The listing builds one solid part. Answer for the finished solid, in the listing's coordinates (mm). Face numbers are marked on the shaded views. Give positions to 0.01 mm unless a question says otherwise; leave off trailing zeros. Write each loop counter-clockwise with the first axis right and the second up, starting at its lowest first coordinate (ties: lowest second). Pieces come first, ordered by that corner, then holes. Notation, with made-up numbers: (-32.5, -29) - (20.5, -29) arc R18 ccw to (20.5, -2) - close; hole circle Ø10 at (8.5, 36). An arc over 180 degrees is marked (long way). Use a Markdown table: item, result. Add a question column.
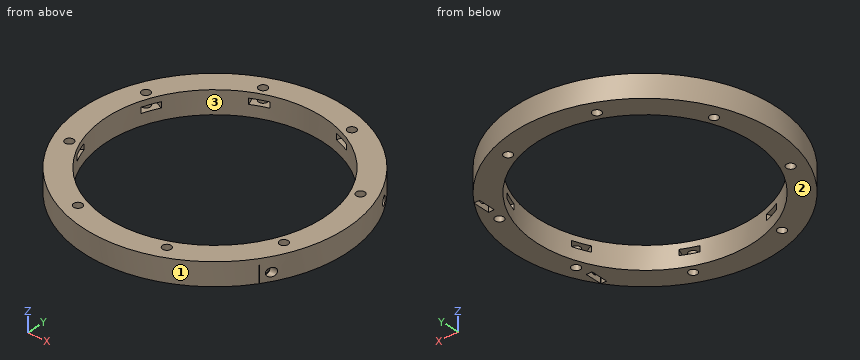
from build123d import *

# Parameters (mm, degrees)
CYLINDER1274_R               = 1.5
CYLINDER1274_DEPTH           = 60
CYLINDER1276_R               = 1.5
CYLINDER1276_DEPTH           = 60
CYLINDER1273_R               = 1.5
CYLINDER1273_DEPTH           = 60
CYLINDER1275_R               = 1.5
CYLINDER1275_DEPTH           = 60
BOX543_W                     = 2
BOX543_H                     = 6
BOX543_DEPTH                 = 6
BOX542_W                     = 2
BOX542_H                     = 6
BOX542_DEPTH                 = 6
BOX541_W                     = 2
BOX541_H                     = 6
BOX541_DEPTH                 = 6
BOX540_W                     = 2
BOX540_H                     = 6
BOX540_DEPTH                 = 6
BOX533_W                     = 8
BOX533_H                     = 6
BOX533_DEPTH                 = 2
BOX539_W                     = 8
BOX539_H                     = 6
BOX539_DEPTH                 = 2
BOX539_PLACEMENT_ANGLE       = 135
BOX534_W                     = 8
BOX534_H                     = 6
BOX534_DEPTH                 = 2
BOX536_W                     = 8
BOX536_H                     = 6
BOX536_DEPTH                 = 2
BOX536_PLACEMENT_ANGLE       = 225
BOX537_W                     = 8
BOX537_H                     = 6
BOX537_DEPTH                 = 2
BOX538_W                     = 8
BOX538_H                     = 6
BOX538_DEPTH                 = 2
BOX538_PLACEMENT_ANGLE       = 45
BOX532_W                     = 8
BOX532_H                     = 6
BOX532_DEPTH                 = 2
BOX535_W                     = 8
BOX535_H                     = 6
BOX535_DEPTH                 = 2
BOX535_PLACEMENT_ANGLE       = 45
COMPOUND921_PLACEMENT_ANGLE  = 22.5
CYLINDER1272_R               = 1.5
CYLINDER1272_DEPTH           = 60
CYLINDER1271_R               = 1.5
CYLINDER1271_DEPTH           = 60
CYLINDER1271_PLACEMENT_ANGLE = 135
CYLINDER1266_R               = 1.5
CYLINDER1266_DEPTH           = 60
CYLINDER1267_R               = 1.5
CYLINDER1267_DEPTH           = 60
CYLINDER1267_PLACEMENT_ANGLE = 225
CYLINDER1270_R               = 1.5
CYLINDER1270_DEPTH           = 60
CYLINDER1268_R               = 1.5
CYLINDER1268_DEPTH           = 60
CYLINDER1268_PLACEMENT_ANGLE = 45
CYLINDER1265_R               = 1.5
CYLINDER1265_DEPTH           = 60
CYLINDER1269_R               = 1.5
CYLINDER1269_DEPTH           = 60
CYLINDER1269_PLACEMENT_ANGLE = 45
COMPOUND919_PLACEMENT_ANGLE  = 22.5
TUBE112_R                    = 46
TUBE112_R_2                  = 38
TUBE112_DEPTH                = 8


with BuildPart() as obj1:
    # Cylinder1274 → Cylinder1274 (new body)
    with BuildSketch(Plane(origin=(32, -23, -5), x_dir=(0, 0, -1), z_dir=(1, 0, 0))):
        Circle(CYLINDER1274_R)
    extrude(amount=CYLINDER1274_DEPTH)


with BuildPart() as obj2:
    # Cylinder1276 → Cylinder1276 (new body)
    with BuildSketch(Plane(origin=(28, 51, 7), x_dir=(0, 0, -1), z_dir=(1, 0, 0))):
        Circle(CYLINDER1276_R)
    extrude(amount=CYLINDER1276_DEPTH)


with BuildPart() as obj3:
    # Cylinder1273 → Cylinder1273 (new body)
    with BuildSketch(Plane(origin=(28, -51, 7), x_dir=(0, 0, -1), z_dir=(1, 0, 0))):
        Circle(CYLINDER1273_R)
    extrude(amount=CYLINDER1273_DEPTH)


with BuildPart() as compound920:
    # Cylinder1275 → Cylinder1275 (new body)
    with BuildSketch(Plane(origin=(32, 23, -5), x_dir=(0, 0, -1), z_dir=(1, 0, 0))):
        Circle(CYLINDER1275_R)
    extrude(amount=CYLINDER1275_DEPTH)

    # Compound920: union obj1, obj2, obj3
    add(obj1.part)
    add(obj2.part)
    add(obj3.part)


with BuildPart() as krychle543:
    # Box543 → Box543 (new body)
    with BuildSketch(Plane(origin=(36, -26, -8), x_dir=(1, 0, 0), z_dir=(0, 0, 1))):
        with Locations((1, 3)):
            Rectangle(BOX543_W, BOX543_H)
    extrude(amount=BOX543_DEPTH)


with BuildPart() as krychle542:
    # Box542 → Box542 (new body)
    with BuildSketch(Plane(origin=(32, 48, 4), x_dir=(1, 0, 0), z_dir=(0, 0, 1))):
        with Locations((1, 3)):
            Rectangle(BOX542_W, BOX542_H)
    extrude(amount=BOX542_DEPTH)


with BuildPart() as krychle541:
    # Box541 → Box541 (new body)
    with BuildSketch(Plane(origin=(32, -54, 4), x_dir=(1, 0, 0), z_dir=(0, 0, 1))):
        with Locations((1, 3)):
            Rectangle(BOX541_W, BOX541_H)
    extrude(amount=BOX541_DEPTH)


with BuildPart() as compound922:
    # Box540 → Box540 (new body)
    with BuildSketch(Plane(origin=(36, 20, -8), x_dir=(1, 0, 0), z_dir=(0, 0, 1))):
        with Locations((1, 3)):
            Rectangle(BOX540_W, BOX540_H)
    extrude(amount=BOX540_DEPTH)

    # Compound922: union Krychle543, Krychle542, Krychle541
    add(krychle543.part)
    add(krychle542.part)
    add(krychle541.part)


with BuildPart() as krychle533:
    # Box533 → Box533 (new body)
    with BuildSketch(Plane(origin=(3, 37, -4), x_dir=(0, 1, 0), z_dir=(0, 0, 1))):
        with Locations((4, 3)):
            Rectangle(BOX533_W, BOX533_H)
    extrude(amount=BOX533_DEPTH)


with BuildPart() as krychle539:
    # Box539 → Box539 (new body)
    with BuildSketch(Plane.XY):
        with Locations((4, 3)):
            Rectangle(BOX539_W, BOX539_H)
    extrude(amount=BOX539_DEPTH)


with BuildPart() as krychle539_1:
    # Box539 placement: moved
    add(krychle539.part.moved(Location((-24.041631, 28.284271, -4))).rotate(Axis((-24.041631, 28.284271, -4), (0, 0, 1)), BOX539_PLACEMENT_ANGLE))


with BuildPart() as krychle534:
    # Box534 → Box534 (new body)
    with BuildSketch(Plane(origin=(-37, 3, -4), x_dir=(-1, 0, 0), z_dir=(0, 0, 1))):
        with Locations((4, 3)):
            Rectangle(BOX534_W, BOX534_H)
    extrude(amount=BOX534_DEPTH)


with BuildPart() as krychle536:
    # Box536 → Box536 (new body)
    with BuildSketch(Plane.XY):
        with Locations((4, 3)):
            Rectangle(BOX536_W, BOX536_H)
    extrude(amount=BOX536_DEPTH)


with BuildPart() as krychle536_1:
    # Box536 placement: moved
    add(krychle536.part.moved(Location((-28.284271, -24.041631, -4))).rotate(Axis((-28.284271, -24.041631, -4), (0, 0, 1)), BOX536_PLACEMENT_ANGLE))


with BuildPart() as krychle537:
    # Box537 → Box537 (new body)
    with BuildSketch(Plane(origin=(-3, -37, -4), x_dir=(0, -1, 0), z_dir=(0, 0, 1))):
        with Locations((4, 3)):
            Rectangle(BOX537_W, BOX537_H)
    extrude(amount=BOX537_DEPTH)


with BuildPart() as krychle538:
    # Box538 → Box538 (new body)
    with BuildSketch(Plane.XY):
        with Locations((4, 3)):
            Rectangle(BOX538_W, BOX538_H)
    extrude(amount=BOX538_DEPTH)


with BuildPart() as krychle538_1:
    # Box538 placement: moved
    add(krychle538.part.moved(Location((24.041631, -28.284271, -4))).rotate(Axis((24.041631, -28.284271, -4), (0, 0, -1)), BOX538_PLACEMENT_ANGLE))


with BuildPart() as krychle532:
    # Box532 → Box532 (new body)
    with BuildSketch(Plane(origin=(37, -3, -4), x_dir=(1, 0, 0), z_dir=(0, 0, 1))):
        with Locations((4, 3)):
            Rectangle(BOX532_W, BOX532_H)
    extrude(amount=BOX532_DEPTH)


with BuildPart() as compound921:
    # Box535 → Box535 (new body)
    with BuildSketch(Plane.XY):
        with Locations((4, 3)):
            Rectangle(BOX535_W, BOX535_H)
    extrude(amount=BOX535_DEPTH)


with BuildPart() as compound921_1:
    # Box535 placement: moved
    add(compound921.part.moved(Location((28.284271, 24.041631, -4))).rotate(Axis((28.284271, 24.041631, -4), (0, 0, 1)), BOX535_PLACEMENT_ANGLE))

    # Compound921: union Krychle533, Krychle539, Krychle534, Krychle536, Krychle537, Krychle538, Krychle532
    add(krychle533.part)
    add(krychle539_1.part)
    add(krychle534.part)
    add(krychle536_1.part)
    add(krychle537.part)
    add(krychle538_1.part)
    add(krychle532.part)


with BuildPart() as compound921_2:
    # Compound921 placement: moved
    add(compound921_1.part.rotate(Axis((0, 0, 0), (0, 0, 1)), COMPOUND921_PLACEMENT_ANGLE))


with BuildPart() as obj4:
    # Cylinder1272 → Cylinder1272 (new body)
    with BuildSketch(Plane(origin=(0, 41, -54), x_dir=(0, 1, 0), z_dir=(0, 0, 1))):
        Circle(CYLINDER1272_R)
    extrude(amount=CYLINDER1272_DEPTH)


with BuildPart() as obj5:
    # Cylinder1271 → Cylinder1271 (new body)
    with BuildSketch(Plane.XY):
        Circle(CYLINDER1271_R)
    extrude(amount=CYLINDER1271_DEPTH)


with BuildPart() as obj5_1:
    # Cylinder1271 placement: moved
    add(obj5.part.moved(Location((-28.991378, 28.991378, -54))).rotate(Axis((-28.991378, 28.991378, -54), (0, 0, 1)), CYLINDER1271_PLACEMENT_ANGLE))


with BuildPart() as obj6:
    # Cylinder1266 → Cylinder1266 (new body)
    with BuildSketch(Plane(origin=(-41, 0, -54), x_dir=(-1, 0, 0), z_dir=(0, 0, 1))):
        Circle(CYLINDER1266_R)
    extrude(amount=CYLINDER1266_DEPTH)


with BuildPart() as obj7:
    # Cylinder1267 → Cylinder1267 (new body)
    with BuildSketch(Plane.XY):
        Circle(CYLINDER1267_R)
    extrude(amount=CYLINDER1267_DEPTH)


with BuildPart() as obj7_1:
    # Cylinder1267 placement: moved
    add(obj7.part.moved(Location((-28.991378, -28.991378, -54))).rotate(Axis((-28.991378, -28.991378, -54), (0, 0, 1)), CYLINDER1267_PLACEMENT_ANGLE))


with BuildPart() as obj8:
    # Cylinder1270 → Cylinder1270 (new body)
    with BuildSketch(Plane(origin=(0, -41, -54), x_dir=(0, -1, 0), z_dir=(0, 0, 1))):
        Circle(CYLINDER1270_R)
    extrude(amount=CYLINDER1270_DEPTH)


with BuildPart() as obj9:
    # Cylinder1268 → Cylinder1268 (new body)
    with BuildSketch(Plane.XY):
        Circle(CYLINDER1268_R)
    extrude(amount=CYLINDER1268_DEPTH)


with BuildPart() as obj9_1:
    # Cylinder1268 placement: moved
    add(obj9.part.moved(Location((28.991378, -28.991378, -54))).rotate(Axis((28.991378, -28.991378, -54), (0, 0, -1)), CYLINDER1268_PLACEMENT_ANGLE))


with BuildPart() as obj10:
    # Cylinder1265 → Cylinder1265 (new body)
    with BuildSketch(Plane(origin=(41, 0, -54), x_dir=(1, 0, 0), z_dir=(0, 0, 1))):
        Circle(CYLINDER1265_R)
    extrude(amount=CYLINDER1265_DEPTH)


with BuildPart() as compound919:
    # Cylinder1269 → Cylinder1269 (new body)
    with BuildSketch(Plane.XY):
        Circle(CYLINDER1269_R)
    extrude(amount=CYLINDER1269_DEPTH)


with BuildPart() as compound919_1:
    # Cylinder1269 placement: moved
    add(compound919.part.moved(Location((28.991378, 28.991378, -54))).rotate(Axis((28.991378, 28.991378, -54), (0, 0, 1)), CYLINDER1269_PLACEMENT_ANGLE))

    # Compound919: union obj4, obj5, obj6, obj7, obj8, obj9, obj10
    add(obj4.part)
    add(obj5_1.part)
    add(obj6.part)
    add(obj7_1.part)
    add(obj8.part)
    add(obj9_1.part)
    add(obj10.part)


with BuildPart() as compound919_2:
    # Compound919 placement: moved
    add(compound919_1.part.rotate(Axis((0, 0, 0), (0, 0, 1)), COMPOUND919_PLACEMENT_ANGLE))


with BuildPart() as cut464:
    # Tube112 → Tube112 (new body)
    with BuildSketch(Plane.XY.offset(-8)):
        Circle(TUBE112_R)
        Circle(TUBE112_R_2, mode=Mode.SUBTRACT)
    extrude(amount=TUBE112_DEPTH)

    # Cut461: cut Compound919
    add(compound919_2.part, mode=Mode.SUBTRACT)

    # Cut462: cut Compound921
    add(compound921_2.part, mode=Mode.SUBTRACT)

    # Cut463: cut Compound922
    add(compound922.part, mode=Mode.SUBTRACT)

    # Cut464: cut Compound920
    add(compound920.part, mode=Mode.SUBTRACT)


solid = cut464.part
1. The part is cut by section A-A (y = 0). Give the vertices of the cut face in (x, z), and give its area (3 significant figures).
2. Given P1, Ø3.5, axis at x = -15.69, y = -37.88, coming from the -Z side; P2, Ø2.5, axis at x = -37.88, y = 15.69, coming from the +Z side; P3, Ø2, axis at x = 37.5, z = -4.5, coming from the +Y side; P4, Ø1, axis at x = 37, y = -22, coming from the -Z side, each flat-ended and moving along its own axis, determine where each tip first touches the part or whether it passes through.
3. For a pull along X with two mould halves and no side action, classify the marked faces 1, 2 and 3 as released by +X, released by -X, zero draft, split by the parting line, or undercut.
4. Consider L1, parallel to Y at x = 33, z = -5.5; L2, parallel to Y at x = 0.5, z = -5.25; L3, parallel to X at y = -39, z = -4.75. Determine where each line is inside the solid, lowest interval first. Write a range as [from, to].
5. The part is cut by section C-C (y = 23). Give the vertices of the cut face in (x, z).
Check values:
| question | item | result |
|---|---|---|
| 1 | outline | (-46, -8) - (-38, -8) - (-38, 0) - (-46, 0) - close; (38, -8) - (46, -8) - (46, 0) - (38, 0) - close |
| 1 | area | 128 mm2 |
| 2 | P1 | stops at z = -8 |
| 2 | P2 | passes through |
| 2 | P3 | stops at y = 28 |
| 2 | P4 | stops at z = -2 |
| 3 | face 1 | split by the parting line |
| 3 | face 2 | zero draft |
| 3 | face 3 | undercut |
| 4 | L1 | y = [-32.05, -24.41], [-21.59, -18.84], [18.84, 21.59], [24.41, 32.05] |
| 4 | L2 | y = [-46, -38], [38, 46] |
| 4 | L3 | x = [-24.39, -16.69], [-14.69, 14.69], [16.69, 24.39] |
| 5 | outline | (-39.84, -8) - (-30.25, -8) - (-30.25, 0) - (-39.84, 0) - close; (30.25, -8) - (36, -8) - (36, -6.5) - (32, -6.5) - (32, -3.5) - (36, -3.5) - (36, -2) - (38, -2) - (38, -3.5) - (39.84, -3.5) - (39.84, 0) - (30.25, 0) - close; (38, -8) - (39.84, -8) - (39.84, -6.5) - (38, -6.5) - close |
